from build123d import *

# Parameters (mm, degrees)
EXTRUDE_1_DEPTH     = 1.25
SKETCH_2_R          = 0.6
CUT_EXTRUDE_1_DEPTH = 3.5
CHAMFER_2_SIZE      = 2
FILLET_1_R          = 1
CHAMFER_3_SIZE      = 5


with BuildPart() as part:
    # 草图1 → 凸台-拉伸1 (new body, symmetric)
    with BuildSketch(Plane(origin=(0, 0, 0), x_dir=(1, 0, 0), z_dir=(0, 1, 0))):
        Polygon((-25, 12.5), (0, 12.5), (10, 22.5), (25, 22.5), (25, -12.5), (-25, -12.5), (-25, -7.5), (-22.025, -7.5), (-22.025, -3.5), (-25.025, -3.5), (-25.025, 3.5), (-22.025, 3.5), (-22.025, 7.5), (-25, 7.5), align=None)
        Polygon((-1.975, -3.5), (-1.975, -7.5), (4.125, -7.5), (4.125, 7.5), (-1.975, 7.5), (-1.975, 3.5), (1.025, 3.5), (1.025, -3.5), align=None, mode=Mode.SUBTRACT)
    extrude(amount=EXTRUDE_1_DEPTH, both=True)

    # 草图2 → 切除-拉伸1 (cut, through all)
    with BuildSketch(Plane(origin=(0, 1.25, 0), x_dir=(1, 0, 0), z_dir=(0, 1, 0))):
        with Locations((-22.025, 4.1)):
            Circle(SKETCH_2_R)
        with Locations((-22.625, 7.5)):
            Circle(SKETCH_2_R)
        with Locations((-22.625, -7.5)):
            Circle(SKETCH_2_R)
        with Locations((-22.025, -4.1)):
            Circle(SKETCH_2_R)
        with Locations((-1.975, 4.1)):
            Circle(SKETCH_2_R)
        with Locations((-1.375, 7.5)):
            Circle(SKETCH_2_R)
        with Locations((-1.375, -7.5)):
            Circle(SKETCH_2_R)
        with Locations((-1.975, -4.1)):
            Circle(SKETCH_2_R)
        with Locations((4.125, -6.9)):
            Circle(SKETCH_2_R)
        with Locations((4.125, 6.9)):
            Circle(SKETCH_2_R)
    extrude(amount=-CUT_EXTRUDE_1_DEPTH, mode=Mode.SUBTRACT)

    # 倒角2
    chamfer_2_edges = [part.edges().sort_by_distance(p)[0] for p in [
        (-25, 0, -12.5),
        (-25, 0, 12.5),
    ]]
    chamfer(chamfer_2_edges, length=CHAMFER_2_SIZE)

    # 圆角1
    fillet_1_edges = [part.edges().sort_by_distance(p)[0] for p in [
        (0, 0, -12.5),
    ]]
    fillet(fillet_1_edges, radius=FILLET_1_R)

    # 倒角3
    chamfer_3_edges = [part.edges().sort_by_distance(p)[0] for p in [
        (25, 0, -22.5),
        (25, 0, 12.5),
    ]]
    chamfer(chamfer_3_edges, length=CHAMFER_3_SIZE)


solid = part.part
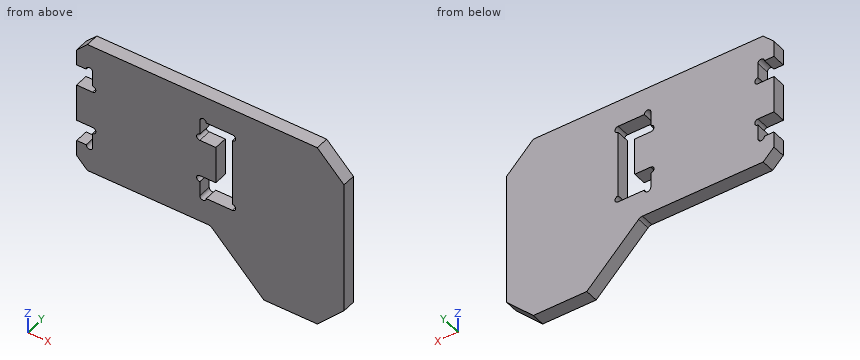
CAD build for the part. Positions are in the model's coordinates, mm. Round coordinates to 2 decimals unless told otherwise and drop trailing zeros. Write each loop counter-clockwise with the first axis right and the second up, starting at its lowest first coordinate (ties: lowest second). Pieces come first, ordered by that corner, then holes. Notation, with made-up numbers: M 11.5,18 L 45.5,18 A20 ccw 45.5,32 Z; hole C -19.75,59.25 d4. An arc over 180 degrees is marked long. Put each result on its own line as item: value. Start each with the question number.
1) Drill centre lines: probe 1 along X at (y, z) = (-0.05, -5) (3 decimals); probe 2 along X at (y, z) = (0.1, 2) (3 decimals); probe 3 along Z at (x, y) = (-0.5, 0.7). Where is each one in solid material? Low to high. Write a range as [from, to].
2) Pin check, flat tips, straight feed: pin 1 Ø0.9 at (x, y) = (-24, -0.5) entering from +Z; pin 2 Ø0.8 at (x, y) = (-23.5, -0.5) entering from -Z; pin 3 Ø1.2 at (x, y) = (-8, -0.5) entering from -Z. Stop position of each tip, or through.
3) Saw through at B-B, the plane x = 21. Write the cut outline in (y, z).
4) Saw through at C-C, the plane x = -14.5. Write the cut outline in (y, z).
5) Saw through at A-A, the plane z = 4.1. Write the cut outline in (x, y) (3 decimals), and give its area (3 significant figures).
Resolved:
1. probe 1: [-22.025, -1.975], [4.125, 25]
1. probe 2: [-25.025, 1.025], [4.125, 25]
1. probe 3: [-12.5, -7.5], [-3.5, 3.5], [7.5, 12.5]
2. pin 1: z = 11.95
2. pin 2: z = -12.4
2. pin 3: z = -12.5
3. outline: M -1.25,-21.5 L 1.25,-21.5 L 1.25,11.5 L -1.25,11.5 Z
4. outline: M -1.25,-12.5 L 1.25,-12.5 L 1.25,12.5 L -1.25,12.5 Z
5. outline: M -21.425,-1.25 L -2.575,-1.25 L -2.575,1.25 L -21.425,1.25 Z; M 4.125,-1.25 L 25,-1.25 L 25,1.25 L 4.125,1.25 Z
5. area: 99.3 mm²
